from build123d import *

# Parameters (mm, degrees)
BOSS_EXTRUDE1_DEPTH = 8.2
SHELL1_T            = -1.5
SKETCH2_W           = 8.2
SKETCH2_H           = 8.2
BOSS_EXTRUDE2_DEPTH = 11.8
SHELL2_START        = -11.8
SHELL2_OUTLINE_W    = 5.2
SHELL2_OUTLINE_H    = 5.2
SHELL2_DEPTH        = 11.8


# Read off the part's stored shape, not the designer's step: Shell2
with BuildPart() as part:
    # Sketch1 → Boss-Extrude1 (new body)
    with BuildSketch(Plane(origin=(0, 0, 0), x_dir=(0, 0, -1), z_dir=(1, 0, 0))):
        Polygon((0, 10), (0, -10), (8.2, -10), (8.2, -4.1), (20, -4.1), (20, 4.1), (8.2, 4.1), (8.2, 10), align=None)
    extrude(amount=BOSS_EXTRUDE1_DEPTH)

    # Shell1
    shell1_openings = [part.faces().sort_by_distance(p)[0] for p in [
        (4.1, -10, -4.1),
        (4.1, 10, -4.1),
        (4.1, 0, -20),
    ]]
    offset(amount=SHELL1_T, openings=shell1_openings, kind=Kind.INTERSECTION)

    # Sketch2 → Boss-Extrude2 (add)
    with BuildSketch(Plane.ZY):
        with Locations((-4.1, 0)):
            Rectangle(SKETCH2_W, SKETCH2_H)
    extrude(amount=BOSS_EXTRUDE2_DEPTH)

    # Shell2 outline → Shell2 (cut)
    with BuildSketch(Plane.YZ.offset(SHELL2_START)):
        with Locations((0, -4.1)):
            Rectangle(SHELL2_OUTLINE_W, SHELL2_OUTLINE_H)
    extrude(amount=SHELL2_DEPTH, mode=Mode.SUBTRACT)


solid = part.part
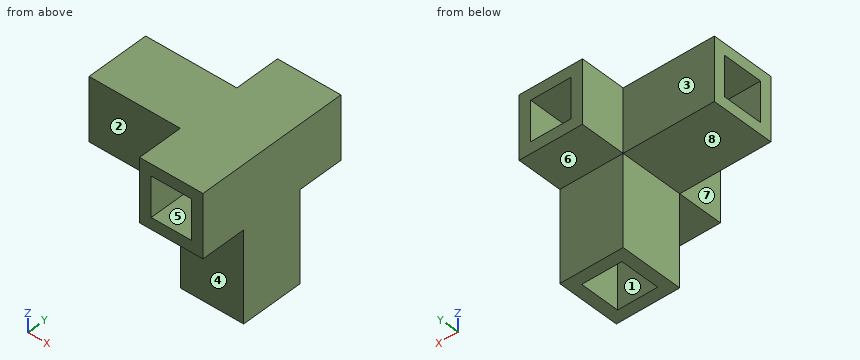
Work out the finished part from the listing and answer in its coordinate system (mm). Face numbers are marked on the shaded views. A direction names the side the tool comes from. Coordinates: 2 decimals unless noted, no trailing zeros. Write each loop counter-clockwise with the first axis right and the second up, starting at its lowest first coordinate (ties: lowest second). Pieces come first, ordered by that corner, then holes. Notation, with made-up numbers: M 29.25,30.5 L 60.25,30.5 A24 ccw 60.25,50.5 Z; hole C 22.5,8 d11. An arc over 180 degrees is marked long. Use one line per item in the form item = value. Start each with the question number.
1. The part is cut by section D-D (y = 3.25). Give the vertices of the cut face in (x, z), plus the area to 3 significant figures.
2. The part is cut by section B-B (x = -6). Give the vertices of the cut face in (y, z), plus the area to 3 significant figures.
3. A tool of negligible diameter and unlimited length cuts with its end or side. For the marked faces 4, 5, 6, 7 and 8, from which of +Z, -Z, +X, -X, +Y, -Y can it reach the whole face along a straight path? Write none if from no direction.
4. The mould has two halves that part along Y. Classify the marked faces 1, 2 and 3: released by +Y, released by -Y, zero draft, split by the parting line, or undercut.
5. Straight lines are drawn through the part: probe 1 along X at (y, z) = (2.5, -12.5); probe 2 along Y at (x, z) = (2, -18); probe 3 along Z at (x, y) = (-2.75, 0). For each, find the intervals that lie inside material, in ascending order. Write a range as from..to.
6. The part is cut by section A-A (z = -5.5). Give the vertices of the cut face in (x, y), plus the area to 3 significant figures.
7. The part is cut by section C-C (x = 5.75). Give the vertices of the cut face in (y, z), plus the area to 3 significant figures.
8. Each of these flat-tipped pins is pushed along its axis until it touches: P1, Ø10, axis at x = -6.5, y = -2, coming from the -Z side; P2, Ø5.5, axis at x = 4, z = -13, coming from the +Y side; P3, Ø2.5, axis at y = -1.5, z = -13, coming from the -X side. Where does it stop, or does it pass through?
Evaluation:
q1.outline = M -11.8,-8.2 L 0,-8.2 L 0,-20 L 8.2,-20 L 8.2,0 L -11.8,0 Z; hole M 1.5,-6.7 L 6.7,-6.7 L 6.7,-1.5 L 1.5,-1.5 Z
q1.area = 234 mm^2
q2.outline = M -4.1,-8.2 L 4.1,-8.2 L 4.1,0 L -4.1,0 Z; hole M -2.6,-6.7 L 2.6,-6.7 L 2.6,-1.5 L -2.6,-1.5 Z
q2.area = 40.2 mm^2
q3.face_4 = -Z, +X, -X, -Y
q3.face_5 = +Y, -Y
q3.face_6 = -Z, +X, -X, +Y
q3.face_7 = +Z, -Z, -X, -Y
q3.face_8 = -Z, -X, +Y, -Y
q4.face_1 = undercut
q4.face_2 = released by -Y
q4.face_3 = released by +Y
q5.probe_1 = 0..1.5, 6.7..8.2
q5.probe_2 = -4.1..-2.6, 2.6..4.1
q5.probe_3 = -8.2..-6.7, -1.5..0
q6.outline = M -11.8,-4.1 L 0,-4.1 L 0,-10 L 1.5,-10 L 1.5,10 L 0,10 L 0,4.1 L -11.8,4.1 L -11.8,2.6 L 0,2.6 L 0,-2.6 L -11.8,-2.6 Z; M 6.7,-10 L 8.2,-10 L 8.2,10 L 6.7,10 Z
q6.area = 95.4 mm^2
q7.outline = M -10,-8.2 L -4.1,-8.2 L -4.1,-20 L -2.6,-20 L -2.6,-6.7 L -10,-6.7 Z; M -10,-1.5 L 10,-1.5 L 10,0 L -10,0 Z; M 2.6,-20 L 4.1,-20 L 4.1,-8.2 L 10,-8.2 L 10,-6.7 L 2.6,-6.7 Z
q7.area = 87.6 mm^2
q8.P1 = -8.2
q8.P2 = 4.1
q8.P3 = 0
